```python
from build123d import *

# Parameters (mm, degrees)
SZKIC1_W                    = 15
SZKIC1_H                    = 30.5
SZKIC1_R                    = 3
DODANIE_WYCI_GNI_CIE1_DEPTH = 2
SZKIC2_R                    = 7.5
DODANIE_WYCI_GNI_CIE2_DEPTH = 6
DODANIE_WYCI_GNI_CIE3_START = -8
SZKIC2_2_R                  = 7.5
DODANIE_WYCI_GNI_CIE3_DEPTH = 6


with BuildPart() as part:
    # Szkic1 → Dodanie-wyciągnięcie1 (new body)
    with BuildSketch(Plane.XY):
        Rectangle(SZKIC1_W, SZKIC1_H)
        with Locations((0, -9.25)):
            Circle(SZKIC1_R, mode=Mode.SUBTRACT)
        with Locations((0, -1.25)):
            Circle(SZKIC1_R, mode=Mode.SUBTRACT)
    extrude(amount=DODANIE_WYCI_GNI_CIE1_DEPTH)

    # Szkic2 → Dodanie-wyciągnięcie2 (add)
    with BuildSketch(Plane.XY.offset(2)):
        with Locations((0, 15.25)):
            Circle(SZKIC2_R)
    extrude(amount=DODANIE_WYCI_GNI_CIE2_DEPTH)

    # Szkic2<2> → Dodanie-wyciągnięcie3 (add)
    with BuildSketch(Plane.XY.offset(2).offset(DODANIE_WYCI_GNI_CIE3_START)):
        with Locations((0, 15.25)):
            Circle(SZKIC2_2_R)
    extrude(amount=DODANIE_WYCI_GNI_CIE3_DEPTH)


solid = part.part
```
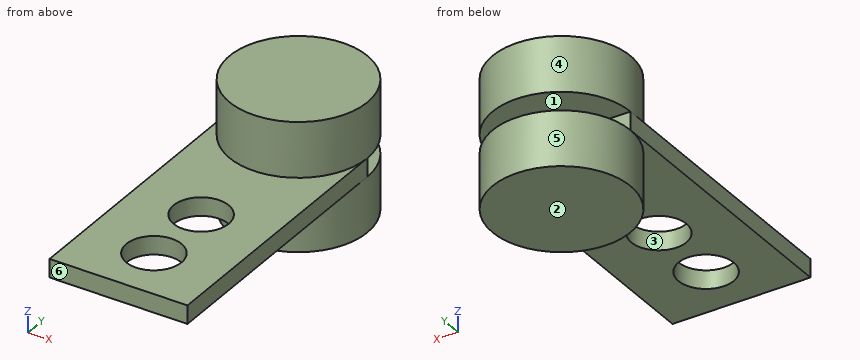
Source: CAD feature listing. Evaluate the final solid. Frame: model axes, mm. Face numbers are marked on the shaded views. A direction names the side the tool comes from. Give positions to 0.01 mm unless a question says otherwise; leave off trailing zeros. Order: outer loops, then holes, each group sorted by start corner. A loop starts at its lowest first (then second) coordinate and runs counter-clockwise, first axis right, second up.
(1) Access query for the marked faces 4, 5 and 6. Directions: +Z, -Z, +X, -X, +Y, -Y. A direction counts if a zero-diameter tool reaches every point of the face in a straight line with its end or side. Return the directions, or none.
(2) Section query C-C (z = 1). Return the cut outline in (x, y), plus the area to 3 significant figures.
(3) Section query B-B (y = -1.25). Return the cut outline in (x, z).
(4) Contact query for flat-ended pins moving along their axis: P1, Ø7.5, axis at x = 3, y = 7, coming from the -Z side; P2, Ø1, axis at x = -4, z = -3, coming from the -Y side; P3, Ø3.5, axis at x = 0, y = -9.25, coming from the -Z side; P4, Ø1.5, axis at x = 2.5, z = -4.5, coming from the +Y side. Output: stop coordinate, or through.
(5) Section query D-D (y = 19). Return the cut outline in (x, z), plus the area to 3 significant figures.
(6) Pull-direction query (Z, two-part tool) for the marked faces 1, 2 and 3; classes: +Z half, -Z half, draft (parallel to the pull), parting line (faces both ways), or undercut.
(7) Section query A-A (x = 0). Return the cut outline in (y, z).
(8) Material intervals for line 1 along Y through (x, z) = (0, 0.4); line 2 along Z through (x, y) = (-1, 18.5); line 3 along Y through (x, z) = (-4, 1.5), sorted ascending.
Outcome:
1. face 4: +Z
1. face 5: -Z
1. face 6: +Z, -Z, +X, -X, -Y
2. outline: (-7.5, -15.25) - (7.5, -15.25) - (7.5, 15.25) - (-7.5, 15.25) - close; hole circle Ø6 at (0, -9.25); hole circle Ø6 at (0, -1.25)
2. area: 401 mm2
3. outline: (-7.5, 0) - (-3, 0) - (-3, 2) - (-7.5, 2) - close; (3, 0) - (7.5, 0) - (7.5, 2) - (3, 2) - close
4. P1: stops at z = -6
4. P2: stops at y = 8.62
4. P3: passes through
4. P4: stops at y = 22.54
5. outline: (-6.5, -6) - (6.5, -6) - (6.5, 0) - (-6.5, 0) - close; (-6.5, 2) - (6.5, 2) - (6.5, 8) - (-6.5, 8) - close
5. area: 156 mm2
6. face 1: undercut
6. face 2: -Z half
6. face 3: draft
7. outline: (-15.25, 0) - (-12.25, 0) - (-12.25, 2) - (-15.25, 2) - close; (-6.25, 0) - (-4.25, 0) - (-4.25, 2) - (-6.25, 2) - close; (1.75, 0) - (7.75, 0) - (7.75, -6) - (22.75, -6) - (22.75, 0) - (15.25, 0) - (15.25, 2) - (22.75, 2) - (22.75, 8) - (7.75, 8) - (7.75, 2) - (1.75, 2) - close
8. line 1: y = -15.25 to -12.25, -6.25 to -4.25, 1.75 to 15.25
8. line 2: z = -6 to 0, 2 to 8
8. line 3: y = -15.25 to 15.25
